```python
from build123d import *

# Parameters (mm, degrees)
SKETCH_1_R      = 3.45
SKETCH_1_R_2    = 2.425
EXTRUDE_1_DEPTH = 3.85
SKETCH_2_R      = 2.425
SKETCH_2_R_2    = 1.25
EXTRUDE_2_DEPTH = 1
SKETCH_3_R      = 0.5
EXTRUDE_3_DEPTH = 1.45


with BuildPart() as part:
    # 草图1 → 凸台-拉伸1 (new body)
    with BuildSketch(Plane(origin=(0, 0, 0), x_dir=(1, 0, 0), z_dir=(0, 1, 0))):
        with Locations(Location((0, 0, 0), (0, 0, 90))):
            Circle(SKETCH_1_R)
        with Locations(Location((0, 0, 0), (0, 0, 90))):
            Circle(SKETCH_1_R_2, mode=Mode.SUBTRACT)
    extrude(amount=EXTRUDE_1_DEPTH)

    # 草图2 → 凸台-拉伸2 (add)
    with BuildSketch(Plane(origin=(0, 1, 0), x_dir=(-1, 0, 0), z_dir=(0, -1, 0))):
        with Locations(Location((0, 0, 0), (0, 0, 90))):
            Circle(SKETCH_2_R)
        with Locations(Location((0, 0, 0), (0, 0, 90))):
            Circle(SKETCH_2_R_2, mode=Mode.SUBTRACT)
    extrude(amount=-EXTRUDE_2_DEPTH)

    # 草图3 → 凸台-拉伸3 (add)
    with BuildSketch(Plane.XZ):
        with BuildLine():
            Line((-14.5, -1.9), (-2.238721733, -2.625))
            ThreePointArc((-2.238721733, -2.625), (-3.45, 0), (-2.238721733, 2.625))
            Line((-2.238721733, 2.625), (-14.5, 1.9))
            ThreePointArc((-14.5, 1.9), (-16.4, 0), (-14.5, -1.9))
        make_face()
        with Locations(Location((-14.5, 0, 0), (0, 0, 270))):
            Circle(SKETCH_3_R, mode=Mode.SUBTRACT)
        with Locations(Location((-12.5, 0, 0), (0, 0, 270))):
            Circle(SKETCH_3_R, mode=Mode.SUBTRACT)
        with Locations(Location((-10.5, 0, 0), (0, 0, 270))):
            Circle(SKETCH_3_R, mode=Mode.SUBTRACT)
        with Locations(Location((-8.5, 0, 0), (0, 0, 270))):
            Circle(SKETCH_3_R, mode=Mode.SUBTRACT)
        with Locations(Location((-6.5, 0, 0), (0, 0, 270))):
            Circle(SKETCH_3_R, mode=Mode.SUBTRACT)
        with Locations(Location((-4.5, 0, 0), (0, 0, 270))):
            Circle(SKETCH_3_R, mode=Mode.SUBTRACT)
    extrude(amount=-EXTRUDE_3_DEPTH)


solid = part.part
```
Can you work these out from the model? Positions are in its coordinate system, mm. A direction names the side the tool comes from. Coordinates: 2 decimals unless noted, no trailing zeros. Loops run counter-clockwise (first coordinate to the right, second up) from the corner with the lowest first, then second, coordinate; pieces in that order, holes last. Notation, with made-up numbers: (70.25, 27) - (88.25, 27) arc R26 cw to (88.25, 55) - close; hole circle Ø11 at (-39.5, -9.5). An arc over 180 degrees is marked (long way). Answer as CSV lines item,"result". Start each with the question number.
1) I need wall thicknesses on line 1 (Y direction, x = -1.5, z = -1.25); line 2 (Z direction, x = -6.25, y = 0.7); line 3 (Y direction, x = -3.25, z = -1.5). Which ranges of each line are inside material? Lowest first, please. Write a range as from..to.
2) Suppose I cut it at C-C (y = 3.25). Please give me the cut outline in (x, z) (3 decimals).
3) Suppose I cut it at A-A (x = 0). Please give me the cut outline in (y, z) (3 decimals).
4) Which directions (+Z, -Z, +X, -X, +Y, -Y) give clear straight access to the entire face, cutting with the end or side of a thin tool? Please do faces 1 (the cylindrical face through (-0.728, 2.912, -2.313)), 2 (the cylindrical face through (-0.728, 0.493, -2.313)), 3 (the flat face through (-7, 0, 1)).
5) Thinking about a two-plate mould opening in Z: for faces 4 (the cylindrical face through (-14, 1, 0)), 5 (the flat face through (-9.4, 1.45, 0)), 6 (the flat face through (-8.455, 0.715, -2.257)), 7 (the cylindrical face through (-4, 1, 0)), which applies, pulls with the +Z half, pulls with the -Z half, needs draft (parallel to the pull), parting line crosses it, or undercut?
6) For pin 1 (1.5 mm diameter, centred on x = 0, z = 0, fed in from +Y) (3 decimals); pin 2 (2 mm diameter, centred on x = -14, z = 2, fed in from -Y); pin 3 (1.5 mm diameter, centred on y = 1, z = 2, fed in from +X); pin 4 (4 mm diameter, centred on x = 0, z = 0, fed in from -Y), each with a flat end and sliding along its axis, tell me the tip position at first contact or that it passes through.
7) Suppose I cut it at D-D (z = 0). Count the separate pieces of the cut face and the enclosed holes in it, plus the area to 3 significant figures.
8) Suppose I cut it at B-B (z = 0.75). Please give me the cut outline in (x, y), plus the area to 3 significant figures.
Check result:
1,line 1,"y = 1..2"
1,line 2,"z = -2.39..-0.43, 0.43..2.39"
1,line 3,"y = 0..1.45"
2,outline,"circle Ø6.9 at (0, 0); hole circle Ø4.85 at (0, 0)"
3,outline,"(0, -3.45) - (3.85, -3.45) - (3.85, -2.425) - (2, -2.425) - (2, -1.25) - (1, -1.25) - (1, -2.425) - (0, -2.425) - close; (0, 2.425) - (1, 2.425) - (1, 1.25) - (2, 1.25) - (2, 2.425) - (3.85, 2.425) - (3.85, 3.45) - (0, 3.45) - close"
4,face 1,"+Y"
4,face 2,"-Y"
4,face 3,"+Z, -Z, +X, -X, -Y"
5,face 4,"undercut"
5,face 5,"needs draft"
5,face 6,"pulls with the -Z half"
5,face 7,"undercut"
6,pin 1,"passes through"
6,pin 2,"stops at y = 0"
6,pin 3,"stops at x = 3.22"
6,pin 4,"stops at y = 1"
7,separate pieces,"8"
7,enclosed holes,"0"
7,area,"20.3 mm²"
8,outline,"(-16.25, 0) - (-2.31, 0) - (-2.31, 1) - (-1, 1) - (-1, 2) - (-2.31, 2) - (-2.31, 3.85) - (-3.37, 3.85) - (-3.37, 1.45) - (-16.25, 1.45) - close; (1, 1) - (2.31, 1) - (2.31, 0) - (3.37, 0) - (3.37, 3.85) - (2.31, 3.85) - (2.31, 2) - (1, 2) - close"
8,area,"29.5 mm²"
